Autodesk Inventor part; units mm, degrees
ref_plane "YZ Plane" through (0, 0, 0) normal (1, 0, 0) x (0, 1, 0)
ref_plane "XZ Plane" through (0, 0, 0) normal (0, 1, 0) x (-1, 0, 0)
ref_plane "XY Plane" through (0, 0, 0) normal (0, 0, 1) x (1, 0, 0)
sketch "Sketch1" plane through (0, 0, 0) normal (0, 0, 1) x (1, 0, 0)
  circle A0 centre (0, 0) radius 20
  line L0 (-35, 35) -> (35, 35)
  line L1 (35, 35) -> (35, -35)
  line L2 (35, -35) -> (-35, -35)
  line L3 (-35, -35) -> (-35, 35)
  line L4 (-35, 35) -> (35, -35) construction
  line L5 (35, 35) -> (-35, -35) construction
  circle A1 centre (-16.35, 16.35) radius 1.6
  circle A2 centre (16.35, 16.35) radius 1.6
  circle A3 centre (-16.35, -16.35) radius 1.6
  circle A4 centre (16.35, -16.35) radius 1.6
  line L6 (35, 5) -> (29, 5)
  line L7 (29, 5) -> (29, -5)
  line L8 (29, -5) -> (35, -5)
  line L9 (35, -5) -> (35, 5)
  line L10 (35, -15) -> (29, -15)
  line L11 (29, -25) -> (35, -25)
  line L12 (29, -15) -> (29, -25)
  line L13 (35, -25) -> (35, -15)
  line L14 (35, 25) -> (29, 25)
  line L15 (29, 15) -> (35, 15)
  line L16 (29, 25) -> (29, 15)
  line L17 (35, 15) -> (35, 25)
  line L18 (35, 5) -> (29, 5)
  line L19 (29, -5) -> (35, -5)
  line L20 (29, 5) -> (29, -5)
  line L21 (35, -5) -> (35, 5)
  line L22 (0, 35) -> (0, -35) construction
  line L23 (-35, 0) -> (35, 0) construction
  line L24 (5, 29) -> (5, 35)
  line L25 (5, 29) -> (5, 35)
  line L26 (-5, 29) -> (5, 29)
  line L27 (5, 35) -> (-5, 35)
  line L28 (15, 29) -> (25, 29)
  line L29 (25, 35) -> (15, 35)
  line L30 (-5, 35) -> (-5, 29)
  line L31 (-5, 35) -> (-5, 29)
  line L32 (25, 29) -> (25, 35)
  line L33 (-5, 29) -> (5, 29)
  line L34 (15, 35) -> (15, 29)
  line L35 (5, 35) -> (-5, 35)
  line L36 (-15, 29) -> (-15, 35)
  line L37 (-25, 35) -> (-25, 29)
  line L38 (-15, 35) -> (-25, 35)
  line L39 (-25, 29) -> (-15, 29)
  line L40 (-29, 5) -> (-35, 5)
  line L41 (-29, 5) -> (-35, 5)
  line L42 (-29, -5) -> (-29, 5)
  line L43 (-35, 5) -> (-35, -5)
  line L44 (-29, 15) -> (-29, 25)
  line L45 (-35, 25) -> (-35, 15)
  line L46 (-35, -5) -> (-29, -5)
  line L47 (-35, -5) -> (-29, -5)
  line L48 (-29, 25) -> (-35, 25)
  line L49 (-29, -5) -> (-29, 5)
  line L50 (-35, 15) -> (-29, 15)
  line L51 (-35, 5) -> (-35, -5)
  line L52 (-29, -15) -> (-35, -15)
  line L53 (-35, -25) -> (-29, -25)
  line L54 (-35, -15) -> (-35, -25)
  line L55 (-29, -25) -> (-29, -15)
  line L56 (-5, -29) -> (-5, -35)
  line L57 (-5, -29) -> (-5, -35)
  line L58 (5, -29) -> (-5, -29)
  line L59 (-5, -35) -> (5, -35)
  line L60 (-15, -29) -> (-25, -29)
  line L61 (-25, -35) -> (-15, -35)
  line L62 (5, -35) -> (5, -29)
  line L63 (5, -35) -> (5, -29)
  line L64 (-25, -29) -> (-25, -35)
  line L65 (5, -29) -> (-5, -29)
  line L66 (-15, -35) -> (-15, -29)
  line L67 (-5, -35) -> (5, -35)
  line L68 (15, -29) -> (15, -35)
  line L69 (25, -35) -> (25, -29)
  line L70 (15, -35) -> (25, -35)
  line L71 (25, -29) -> (15, -29)
  point P0 (29, 0)
  point P1 (29, -20)
  point P2 (35, -20)
  point P3 (29, 20)
  point P4 (35, 20)
  point P5 (29, 0)
  point P6 (0, 29)
  point P7 (20, 35)
  point P8 (20, 29)
  point P9 (0, 29)
  point P10 (0, 35)
  point P11 (0, 35)
  point P12 (-20, 29)
  point P13 (-20, 35)
  point P14 (-29, 0)
  point P15 (-35, 20)
  point P16 (-29, 20)
  point P17 (-29, 0)
  point P18 (-35, 0)
  point P19 (-35, 0)
  point P20 (-29, -20)
  point P21 (-35, -20)
  point P22 (0, -29)
  point P23 (-20, -35)
  point P24 (-20, -29)
  point P25 (0, -29)
  point P26 (0, -35)
  point P27 (0, -35)
  point P28 (20, -29)
  point P29 (20, -35)
  dimension "d0" = 40
  dimension "d1" = 70
  dimension "d2" = 70
  dimension "d3" = 32.7
  dimension "d4" = 3.2
  dimension "d5" = 6
  dimension "d6" = 10
  dimension "d9" = 20
  dimension "d12" = 20
  dimension "d17" = 360
extrude "Extrusion1" add sketch "Sketch1" along normal blind 6 contours L0 L37 L39 L36 L30 L26 L24 L34 L28 L32 L1 L14 L16 L15 L6 L7 L8 L10 L12 L11 L2 L69 L71 L68 L62 L58 L56 L66 L60 L64 L3 L53 L55 L52 L46 L42 L40 L50 L44 L48
equation "\"d9\" = 2 * d6"
equation "\"d12\" = 2 * d6"
equation "\"BendRadius\" = Thickness"
equation "\"BendReliefWidth\" = Thickness"
equation "\"BendReliefDepth\" = 0.5 * Thickness"
equation "\"CornerReliefSize\" = 4 * Thickness"
equation "\"MinimumRemnant\" = 2 * Thickness"
equation "\"TransitionRadius\" = BendRadius"
equation "\"JacobiRadiusSize\" = Thickness"
equation "\"GapSize\" = Thickness"
properties part number "joystick behuizing boevnzijde" material "Wood (Birch)"
Input: part model. Units: mm. Frame: model coordinates. A direction names the side the tool comes from. Give positions to 0.01 mm unless a question says otherwise; leave off trailing zeros. Loops run counter-clockwise (first coordinate to the right, second up) from the corner with the lowest first, then second, coordinate; pieces in that order, holes last. Notation, with made-up numbers: (24, -28) - (29, -28) arc R21 cw to (29, -2) - close; hole circle Ø6 at (31, -11.5). An arc over 180 degrees is marked (long way). Use CSV: the item, a comma, the result in double quotes. Start each with the question number.
Item 1: Reachability of faces 4 (the flat face through (-32, -25, 3)), 5 (the flat face through (25, 32, 3)), 6 (the flat face through (29, 0, 3)), 7 (the flat face through (25, -32, 3)) from +Z, -Z, +X, -X, +Y, -Y: full face, straight path, thin tool, end or side. Return the list, or none.
Item 2: Contact query for flat-ended pins moving along their axis: P1, Ø3, axis at x = 16.35, y = -16.35, coming from the -Z side; P2, Ø3, axis at y = -22.5, z = 3, coming from the +X side; P3, Ø1.8, axis at x = 0, z = 4, coming from the +Y side; P4, Ø8, axis at x = 20.5, y = -5.5, coming from the -Z side. Output: stop coordinate, or through.
Item 3: Mould query, pull axis Y, two halves, no side actions, for faces 1 (the flat face through (-32, -15, 3)), 2 (the flat face through (-35, 10, 3)), 3 (the flat face through (20, -29, 3)). Classes: pulls with the +Y half, pulls with the -Y half, needs draft (parallel to the pull), parting line crosses it, or undercut.
Item 4: Section D-D on z = 2.15. State how many separate pieces and enclosed holes the cut face has, then the cut area to 3 significant figures.
Item 5: Line query: line 1 (X direction, y = 31.5, z = 2.3); line 2 (Y direction, x = 16.35, z = 2.05). Output: solid intervals per line, ascending.
Item 6: Section C-C on y = -16.35. Return loops of the section in (x, z).
Item 7: Section A-A on y = 0. Return loops of the section in (x, z), then the cut area to 3 significant figures.
Ans:
1,face 4,"+Z, -Z, -X"
1,face 5,"+Z, -Z, +Y"
1,face 6,"+Z, -Z, +X"
1,face 7,"+Z, -Z, -Y"
2,P1,"passes through"
2,P2,"stops at x = 29"
2,P3,"stops at y = 29"
2,P4,"stops at z = 0"
3,face 1,"undercut"
3,face 2,"needs draft"
3,face 3,"pulls with the -Y half"
4,separate pieces,"1"
4,enclosed holes,"5"
4,area,"2,890 mm2"
5,line 1,"x = -35 to -25, -15 to -5, 5 to 15, 25 to 35"
5,line 2,"y = -29 to -17.95, -14.75 to -11.52, 11.52 to 14.75, 17.95 to 29"
6,outline,"(-29, 0) - (-17.95, 0) - (-17.95, 6) - (-29, 6) - close; (-14.75, 0) - (-11.52, 0) - (-11.52, 6) - (-14.75, 6) - close; (11.52, 0) - (14.75, 0) - (14.75, 6) - (11.52, 6) - close; (17.95, 0) - (29, 0) - (29, 6) - (17.95, 6) - close"
7,outline,"(-29, 0) - (-20, 0) - (-20, 6) - (-29, 6) - close; (20, 0) - (29, 0) - (29, 6) - (20, 6) - close"
7,area,"108 mm2"
